from build123d import *

# Parameters (mm, degrees)
SKETCH1_R           = 5.824269922
SKETCH1_R_2         = 15.183436718
SKETCH1_R_3         = 2.097724336
SKETCH1_R_4         = 1.501171646
SKETCH1_R_5         = 6.046381911
SKETCH1_R_6         = 1.233955492
SKETCH1_R_7         = 4.738389089
SKETCH1_R_8         = 1.524
BOSS_EXTRUDE1_DEPTH = 12.7
SKETCH3_R           = 14.2875


with BuildPart() as part:
    # Sketch1 → Boss-Extrude1 (new body)
    with BuildSketch(Plane(origin=(0, 0, 0), x_dir=(1, 0, 0), z_dir=(0, 1, 0))):
        with BuildLine():
            Line((181.053619211, 279.591938546), (200.093166842, 279.591938546))
            Line((200.093166842, 279.591938546), (200.093166842, 162.94458344))
            Line((200.093166842, 162.94458344), (645.714984179, 162.94458344))
            Line((645.714984179, 162.94458344), (645.714984179, 267.541591944))
            Line((645.714984179, 267.541591944), (651.459778015, 267.541591944))
            Line((651.459778015, 267.541591944), (659.592709072, 270.588129637))
            Line((659.592709072, 270.588129637), (659.592709072, 310.92735289))
            ThreePointArc((659.592709072, 310.92735289), (662.356769374, 313.691413192), (665.120829676, 310.92735289))
            Line((665.120829676, 310.92735289), (665.120829676, 270.588129637))
            Line((665.120829676, 270.588129637), (673.253760733, 267.541591944))
            Line((673.253760733, 267.541591944), (695.362412179, 267.541591944))
            Line((695.362412179, 267.541591944), (695.362412179, 1184.427811096))
            Line((695.362412179, 1184.427811096), (181.053619211, 1184.427811096))
            Line((181.053619211, 1184.427811096), (181.053619211, 279.591938546))
        make_face()
        with Locations(Location((324.163687625, 333.156445716, 0), (0, 0, 270))):  # turned: the seam where the file's is
            Circle(SKETCH1_R, mode=Mode.SUBTRACT)
        with Locations(Location((498.003337343, 333.156445716, 0), (0, 0, 270))):  # turned: the seam where the file's is
            Circle(SKETCH1_R, mode=Mode.SUBTRACT)
        with Locations(Location((285.454913552, 435.726712451, 0), (0, 0, 270))):  # turned: the seam where the file's is
            Circle(SKETCH1_R, mode=Mode.SUBTRACT)
        with Locations(Location((269.478274819, 494.373532098, 0), (0, 0, 270))):  # turned: the seam where the file's is
            Circle(SKETCH1_R, mode=Mode.SUBTRACT)
        with Locations(Location((283.113483006, 488.0772742, 0), (0, 0, 270))):  # turned: the seam where the file's is
            Circle(SKETCH1_R, mode=Mode.SUBTRACT)
        with Locations(Location((299.283235774, 440.456463852, 0), (0, 0, 270))):  # turned: the seam where the file's is
            Circle(SKETCH1_R, mode=Mode.SUBTRACT)
        with Locations(Location((536.712111416, 435.726712451, 0), (0, 0, 270))):  # turned: the seam where the file's is
            Circle(SKETCH1_R, mode=Mode.SUBTRACT)
        with Locations(Location((552.688750149, 494.373532098, 0), (0, 0, 270))):  # turned: the seam where the file's is
            Circle(SKETCH1_R, mode=Mode.SUBTRACT)
        with Locations(Location((539.053541962, 488.0772742, 0), (0, 0, 270))):  # turned: the seam where the file's is
            Circle(SKETCH1_R, mode=Mode.SUBTRACT)
        with Locations(Location((522.883789195, 440.456463852, 0), (0, 0, 270))):  # turned: the seam where the file's is
            Circle(SKETCH1_R, mode=Mode.SUBTRACT)
        with Locations(Location((594.651015644, 211.880261627, 0), (0, 0, 270))):  # turned: the seam where the file's is
            Circle(SKETCH1_R_2, mode=Mode.SUBTRACT)
        with Locations(Location((221.612450161, 232.383888713, 0), (0, 0, 270))):  # turned: the seam where the file's is
            Circle(SKETCH1_R_3, mode=Mode.SUBTRACT)
        with Locations(Location((221.612450161, 195.241828402, 0), (0, 0, 270))):  # turned: the seam where the file's is
            Circle(SKETCH1_R_3, mode=Mode.SUBTRACT)
        with Locations(Location((633.069124813, 232.383888713, 0), (0, 0, 270))):  # turned: the seam where the file's is
            Circle(SKETCH1_R_3, mode=Mode.SUBTRACT)
        with Locations(Location((633.069124813, 195.241828402, 0), (0, 0, 270))):  # turned: the seam where the file's is
            Circle(SKETCH1_R_3, mode=Mode.SUBTRACT)
        with Locations(Location((402.196528277, 215.362632519, 0), (0, 0, 270))):  # turned: the seam where the file's is
            Circle(SKETCH1_R_4, mode=Mode.SUBTRACT)
        with Locations(Location((438.228028644, 175.135683479, 0), (0, 0, 270))):  # turned: the seam where the file's is
            Circle(SKETCH1_R_4, mode=Mode.SUBTRACT)
        with Locations(Location((477.221022192, 175.135683479, 0), (0, 0, 270))):  # turned: the seam where the file's is
            Circle(SKETCH1_R_4, mode=Mode.SUBTRACT)
        with Locations(Location((454.639636688, 176.863221168, 0), (0, 0, 270))):  # turned: the seam where the file's is
            Circle(SKETCH1_R_5, mode=Mode.SUBTRACT)
        with Locations(Location((225.832143337, 496.894899007, 0), (0, 0, 270))):  # turned: the seam where the file's is
            Circle(SKETCH1_R_6, mode=Mode.SUBTRACT)
        with Locations(Location((236.567556118, 396.296677519, 0), (0, 0, 270))):  # turned: the seam where the file's is
            Circle(SKETCH1_R_6, mode=Mode.SUBTRACT)
        with Locations(Location((269.884354403, 372.851523171, 0), (0, 0, 270))):  # turned: the seam where the file's is
            Circle(SKETCH1_R_6, mode=Mode.SUBTRACT)
        with Locations(Location((304.280863743, 346.938457838, 0), (0, 0, 270))):  # turned: the seam where the file's is
            Circle(SKETCH1_R_6, mode=Mode.SUBTRACT)
        with Locations(Location((596.334881631, 496.894899007, 0), (0, 0, 270))):  # turned: the seam where the file's is
            Circle(SKETCH1_R_6, mode=Mode.SUBTRACT)
        with Locations(Location((585.59946885, 396.296677519, 0), (0, 0, 270))):  # turned: the seam where the file's is
            Circle(SKETCH1_R_6, mode=Mode.SUBTRACT)
        with Locations(Location((552.282670565, 372.851523171, 0), (0, 0, 270))):  # turned: the seam where the file's is
            Circle(SKETCH1_R_6, mode=Mode.SUBTRACT)
        with Locations(Location((517.886161225, 346.938457838, 0), (0, 0, 270))):  # turned: the seam where the file's is
            Circle(SKETCH1_R_6, mode=Mode.SUBTRACT)
        with Locations(Location((217.200519411, 959.83603663, 0), (0, 0, 270))):  # turned: the seam where the file's is
            Circle(SKETCH1_R_7, mode=Mode.SUBTRACT)
        with Locations(Location((251.849989627, 959.83603663, 0), (0, 0, 270))):  # turned: the seam where the file's is
            Circle(SKETCH1_R_7, mode=Mode.SUBTRACT)
        with Locations(Location((272.894732067, 508.643077531, 0), (0, 0, 270))):  # turned: the seam where the file's is
            Circle(SKETCH1_R_8, mode=Mode.SUBTRACT)
        with Locations(Location((268.450589155, 466.396381192, 0), (0, 0, 270))):  # turned: the seam where the file's is
            Circle(SKETCH1_R_8, mode=Mode.SUBTRACT)
        with Locations(Location((271.126563031, 440.408557976, 0), (0, 0, 270))):  # turned: the seam where the file's is
            Circle(SKETCH1_R_8, mode=Mode.SUBTRACT)
        with Locations(Location((304.473314405, 417.292260573, 0), (0, 0, 270))):  # turned: the seam where the file's is
            Circle(SKETCH1_R_8, mode=Mode.SUBTRACT)
        with Locations(Location((549.272292901, 508.643077531, 0), (0, 0, 270))):  # turned: the seam where the file's is
            Circle(SKETCH1_R_8, mode=Mode.SUBTRACT)
        with Locations(Location((553.716435813, 466.396381192, 0), (0, 0, 270))):  # turned: the seam where the file's is
            Circle(SKETCH1_R_8, mode=Mode.SUBTRACT)
        with Locations(Location((551.040461937, 440.408557976, 0), (0, 0, 270))):  # turned: the seam where the file's is
            Circle(SKETCH1_R_8, mode=Mode.SUBTRACT)
        with Locations(Location((517.693710564, 417.292260573, 0), (0, 0, 270))):  # turned: the seam where the file's is
            Circle(SKETCH1_R_8, mode=Mode.SUBTRACT)
        with BuildLine():
            Line((280.043534807, 466.342038413), (292.284373288, 471.080427502))
            ThreePointArc((292.284373288, 471.080427502), (299.818428707, 467.751426271), (296.489427475, 460.217370852))
            Line((296.489427475, 460.217370852), (284.248588994, 455.478981762))
            ThreePointArc((284.248588994, 455.478981762), (276.714533575, 458.807982994), (280.043534807, 466.342038413))
        make_face(mode=Mode.SUBTRACT)
        with BuildLine():
            Line((542.123490162, 466.342038413), (529.882651681, 471.080427502))
            ThreePointArc((529.882651681, 471.080427502), (522.348596262, 467.751426271), (525.677597493, 460.217370852))
            Line((525.677597493, 460.217370852), (537.918435974, 455.478981762))
            ThreePointArc((537.918435974, 455.478981762), (545.452491393, 458.807982994), (542.123490162, 466.342038413))
        make_face(mode=Mode.SUBTRACT)
        with BuildLine():
            Line((209.707710439, 480.9937085), (209.707710439, 447.193199663))
            ThreePointArc((209.707710439, 447.193199663), (207.575435349, 445.060924572), (205.443160259, 447.193199663))
            Line((205.443160259, 447.193199663), (205.443160259, 480.9937085))
            ThreePointArc((205.443160259, 480.9937085), (207.575435349, 483.12598359), (209.707710439, 480.9937085))
        make_face(mode=Mode.SUBTRACT)
        with BuildLine():
            Line((242.244648853, 480.9937085), (242.244648853, 447.193199663))
            ThreePointArc((242.244648853, 447.193199663), (244.376923944, 445.060924572), (246.509199034, 447.193199663))
            Line((246.509199034, 447.193199663), (246.509199034, 480.9937085))
            ThreePointArc((246.509199034, 480.9937085), (244.376923944, 483.12598359), (242.244648853, 480.9937085))
        make_face(mode=Mode.SUBTRACT)
        with BuildLine():
            Line((576.352211687, 480.9937085), (576.352211687, 447.193199663))
            ThreePointArc((576.352211687, 447.193199663), (578.484486777, 445.060924572), (580.616761867, 447.193199663))
            Line((580.616761867, 447.193199663), (580.616761867, 480.9937085))
            ThreePointArc((580.616761867, 480.9937085), (578.484486777, 483.12598359), (576.352211687, 480.9937085))
        make_face(mode=Mode.SUBTRACT)
        with BuildLine():
            Line((613.864458645, 480.9937085), (613.864458645, 447.193199663))
            ThreePointArc((613.864458645, 447.193199663), (615.996733735, 445.060924572), (618.129008825, 447.193199663))
            Line((618.129008825, 447.193199663), (618.129008825, 480.9937085))
            ThreePointArc((618.129008825, 480.9937085), (615.996733735, 483.12598359), (613.864458645, 480.9937085))
        make_face(mode=Mode.SUBTRACT)
        with BuildLine():
            Line((640.619770917, 319.710384153), (640.545012441, 319.844114807))
            ThreePointArc((640.545012441, 319.844114807), (630.971841378, 327.402872478), (618.857738395, 325.978467108))
            Line((618.857738395, 325.978467108), (436.133708882, 223.831579783))
            ThreePointArc((436.133708882, 223.831579783), (433.695399956, 220.743460085), (434.154885559, 216.835684929))
            Line((434.154885559, 216.835684929), (444.765494249, 197.855046105))
            ThreePointArc((444.765494249, 197.855046105), (447.853613947, 195.416737179), (451.761389102, 195.876222782))
            Line((451.761389102, 195.876222782), (634.485418615, 298.023110107))
            ThreePointArc((634.485418615, 298.023110107), (642.044176286, 307.59628117), (640.619770917, 319.710384153))
        make_face(mode=Mode.SUBTRACT)
        with BuildLine():
            Line((235.713447154, 952.32831259), (237.858461253, 950.094878062))
            ThreePointArc((237.858461253, 950.094878062), (243.9998787, 949.970855421), (244.123901341, 956.112272868))
            Line((244.123901341, 956.112272868), (241.978887242, 958.345707396))
            ThreePointArc((241.978887242, 958.345707396), (240.007514596, 965.101257084), (233.337061884, 967.343760669))
            Line((233.337061884, 967.343760669), (231.192047785, 969.577195197))
            ThreePointArc((231.192047785, 969.577195197), (225.050630338, 969.701217838), (224.926607697, 963.559800391))
            Line((224.926607697, 963.559800391), (227.071621796, 961.326365863))
            ThreePointArc((227.071621796, 961.326365863), (229.042994442, 954.570816175), (235.713447154, 952.32831259))
        make_face(mode=Mode.SUBTRACT)
    extrude(amount=BOSS_EXTRUDE1_DEPTH)

    # Cut-Sweep1: sweep along a path in Sketch2
    with BuildLine(Plane(origin=(662.356769374, 0, 0), x_dir=(0, 0, -1), z_dir=(1, 0, 0))) as cut_sweep1_path:
        Line((267.541591944, 12.7), (521.541591944, 17.4625))
    # Sketch3 → Cut-Sweep1 (sweep, cut)
    with BuildSketch(Plane.XY.offset(-267.541591944)):
        with Locations((662.356769374, 22.225)):
            Circle(SKETCH3_R)
    sweep(path=cut_sweep1_path.line, mode=Mode.SUBTRACT)


solid = part.part
Input: part model. Units: mm. Frame: model coordinates. A direction names the side the tool comes from. Coordinates: 2 decimals unless noted, no trailing zeros.
Q1. Material intervals for line 1 (X direction, y = 7.25, z = -950); line 2 (Z direction, x = 458, y = 12.25); line 3 (Z direction, x = 583, y = 9.5), sorted ascending.
Q2. Cut plane A-A (y = 5). Give the number of separate pieces and of enclosed holes in the cut face, then the cut area to 3 significant figures.
Q3. Draft query along Z for faces 3 (the face through (541.84, 6.26, -246.23)), 4 (the face through (435, 12.7, -681)), 5 (the face through (588.836, 6.261, -197.855)). Return one class per face: +Z half, -Z half, draft (parallel to the pull), parting line (faces both ways), or undercut.
Q4. Set-up query: faces 1 (the face through (528.775, 6.261, -275.62)), 2 (the face through (435, 0, -681)). Return all of +Z, -Z, +X, -X, +Y, -Y with unobstructed straight access to the full face (end or side cutting, diameter ignored); none if empty.
Q5. Contact query for flat-ended pins moving along their axis: pin 1 (2.5 mm diameter, centred on x = 438.23, z = -175.14, fed in from +Y); pin 2 (4 mm diameter, centred on y = 4, z = -219, fed in from +X) (3 decimals). Output: stop coordinate, or through.
Working result:
1. line 1: x = 181.05 to 237.95, 244.03 to 695.36
1. line 2: z = -1184.43 to -236.06, -199.36 to -181.89, -171.84 to -162.94
1. line 3: z = -1184.43 to -305.93, -269.24 to -221.62, -202.14 to -162.94
2. separate pieces: 1
2. enclosed holes: 45
2. area: 507,000 mm2
3. face 3: undercut
3. face 4: draft
3. face 5: undercut
4. face 1: +Y, -Y
4. face 2: +Z, -Z, +X, -X, -Y
5. pin 1: passes through
5. pin 2: stops at x = 645.715
